Geometry: final body of the model. Coordinates: model frame, mm. Face numbers are marked on the shaded views. A direction names the side the tool comes from. Round coordinates to 2 decimals unless told otherwise and drop trailing zeros. Loops run counter-clockwise (first coordinate to the right, second up) from the corner with the lowest first, then second, coordinate; pieces in that order, holes last. Notation, with made-up numbers: M 2,27 L 21,27 A21 ccw 21,56 Z; hole C 85,72 d7. An arc over 180 degrees is marked long. Answer as a JSON object with one key per item and string values.
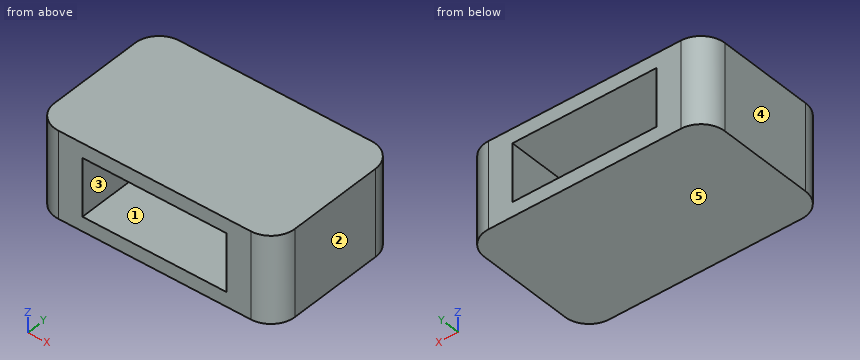
from build123d import *

# Parameters (mm, degrees)
F1_DEPTH = 3
F2_W     = 4
F2_H     = 20
F2_W_2   = 5.5355339059
F3_DEPTH = 7
F4_DEPTH = 5
F5_W     = 4
F5_H     = 20
F6_DEPTH = 3


with BuildPart() as f1:
    # F0 (on Top) → F1 (new body)
    with BuildSketch(Plane.XY):
        with BuildLine():
            Line((-45, 0), (-5, 0))
            ThreePointArc((-5, 0), (-1.4644660941, 1.4644660941), (0, 5))
            Line((0, 5), (0, 25))
            ThreePointArc((0, 25), (-1.4644660941, 28.5355339059), (-5, 30))
            Line((-5, 30), (-45, 30))
            ThreePointArc((-45, 30), (-48.5355339059, 28.5355339059), (-50, 25))
            Line((-50, 25), (-50, 5))
            ThreePointArc((-50, 5), (-48.5355339059, 1.4644660941), (-45, 0))
        make_face()
    extrude(amount=F1_DEPTH)

    # F2 (on face) → F3 (join)
    with BuildSketch(Plane.XY.offset(3)):
        with BuildLine():
            Line((-45, 0), (-40, 0))
            Line((-40, 0), (-40, 30))
            Line((-40, 30), (-45, 30))
            ThreePointArc((-45, 30), (-48.5355339059, 28.5355339059), (-50, 25))
            Line((-50, 25), (-50, 5))
            ThreePointArc((-50, 5), (-48.5355339059, 1.4644660941), (-45, 0))
        make_face()
        with Locations((-45, 15)):
            Rectangle(F2_W, F2_H, mode=Mode.SUBTRACT)
        with BuildLine():
            Line((-10, 0), (-5, 0))
            ThreePointArc((-5, 0), (-1.4644660941, 1.4644660941), (0, 5))
            Line((0, 5), (0, 25))
            ThreePointArc((0, 25), (-1.4644660941, 28.5355339059), (-5, 30))
            Line((-5, 30), (-10, 30))
            Line((-10, 30), (-10, 0))
        make_face()
        with Locations((-4.232233047, 15)):
            Rectangle(F2_W_2, F2_H, mode=Mode.SUBTRACT)
    extrude(amount=F3_DEPTH)

    # F4 (add): faces of the model
    f4_faces = [f1.faces().sort_by_distance(p)[0] for p in [
        (-42.5, 0.316227766, 10),
        (-7.5, 0.316227766, 10),
    ]]
    extrude(f4_faces, amount=F4_DEPTH)

    # F5 (on face) → F6 (join)
    with BuildSketch(Plane.XY.offset(15)):
        with BuildLine():
            Line((-45, 0), (-40, 0))
            Line((-40, 0), (-40, 30))
            Line((-40, 30), (-45, 30))
            ThreePointArc((-45, 30), (-48.5355339059, 28.5355339059), (-50, 25))
            Line((-50, 25), (-50, 5))
            ThreePointArc((-50, 5), (-48.5355339059, 1.4644660941), (-45, 0))
        make_face()
        with Locations((-45, 15)):
            Rectangle(F5_W, F5_H, mode=Mode.SUBTRACT)
        with BuildLine():
            Line((-40, 0), (-5, 0))
            ThreePointArc((-5, 0), (-1.4644660941, 1.4644660941), (0, 5))
            Line((0, 5), (0, 25))
            ThreePointArc((0, 25), (-1.4644660941, 28.5355339059), (-5, 30))
            Line((-5, 30), (-40, 30))
            Line((-40, 30), (-40, 0))
        make_face()
        with Locations((-45, 15)):
            Rectangle(F5_W, F5_H)
    extrude(amount=F6_DEPTH)


solid = f1.part
1) Section query D-D (y = 26.5). Return the cut outline in (x, z), and give its area (3 significant figures).
Results:
{"outline": "M -49.77,0 L -0.23,0 L -0.23,18 L -49.77,18 Z; hole M -40,3 L -10,3 L -10,15 L -40,15 Z", "area": "532 mm2"}
2) Ray query, line 1 (X direction, y = 17.5, z = 7); line 2 (Z direction, x = -15.5, y = 7); line 3 (Y direction, x = -6.5, z = 9). Return the intervals inside material, ascending.
Results:
{"line 1": "-50 to -47, -43 to -40, -10 to -7, -1.46 to 0", "line 2": "0 to 3, 15 to 18", "line 3": "0 to 5, 25 to 30"}
3) Section query C-C (y = 12). Return the cut outline in (x, z).
Results:
{"outline": "M -50,0 L 0,0 L 0,18 L -50,18 Z; hole M -47,3 L -43,3 L -43,15 L -47,15 Z; hole M -40,3 L -10,3 L -10,15 L -40,15 Z; hole M -7,3 L -1.46,3 L -1.46,15 L -7,15 Z"}
4) Pin query (flat end, axial travel): P1, Ø1.2, axis at x = -44.5, z = 10.5, coming from the -Y side; P2, Ø1, axis at y = 3, z = 5.5, coming from the +X side. Return the tip coordinate at first contact, or that it passes through.
Results:
{"P1": "y = 0", "P2": "x = -0.23"}
5) Pull-direction query (Z, two-part tool) for the marked faces 3, 4 and 5; classes: +Z half, -Z half, draft (parallel to the pull), parting line (faces both ways), or undercut.
Results:
{"face 3": "undercut", "face 4": "draft", "face 5": "-Z half"}
6) Section query B-B (x = -16). Return the cut outline in (y, z).
Results:
{"outline": "M 0,0 L 30,0 L 30,3 L 0,3 Z; M 0,15 L 30,15 L 30,18 L 0,18 Z"}
7) Section query A-A (z = 11.75). Return the cut outline in (x, y).
Results:
{"outline": "M -50,5 A5 ccw -45,0 L -40,0 L -40,30 L -45,30 A5 ccw -50,25 Z; M -10,0 L -5,0 A5 ccw 0,5 L 0,25 A5 ccw -5,30 L -10,30 Z; hole M -47,5 L -43,5 L -43,25 L -47,25 Z; hole M -7,5 L -1.46,5 L -1.46,25 L -7,25 Z"}
8) Reachability of the marked faces 1 and 2 from +Z, -Z, +X, -X, +Y, -Y: full face, straight path, thin tool, end or side. Return the list, or none.
Results:
{"face 1": "+Y, -Y", "face 2": "+Z, -Z, +X, +Y, -Y"}
